Could you check a few things on this model? Use its own coordinates, in mm. A direction names the side the tool comes from. Round coordinates to 2 decimals unless told otherwise and drop trailing zeros. Write each loop counter-clockwise with the first axis right and the second up, starting at its lowest first coordinate (ties: lowest second). Pieces come first, ordered by that corner, then holes. Notation, with made-up numbers: M -27.5,77.5 L -16.5,77.5 A11 cw -16.5,92.5 Z; hole C 62.25,65 d2. An arc over 180 degrees is marked long. One line per item, written item: value. Start each with the question number.
(1) I want a section at C-C on z = 46.5. Please give me the cut outline in (x, y), and give its area (3 significant figures).
(2) Thinking about a two-plate mould opening in Y: for faces 1 (the face through (12.535, 4.207, 24.65)), 2 (the face through (60, 14, 25)), 3 (the face through (10, 39.879, 25)), which applies, released by +Y, released by -Y, zero draft, split by the parting line, or undercut?
(3) I want a section at B-B on x = 12. Please give me the cut outline in (y, z), and give its area (3 significant figures).
(4) Which directions (+Z, -Z, +X, -X, +Y, -Y) give clear straight access to the entire face, cutting with the end or side of a thin tool? Please do faces 4 (the face through (39.93, 34.845, 24.719)), 5 (the face through (7, 8.151, 25)), 6 (the face through (47.535, 4.404, 24.65)).
(5) I want a section at A-A on y = 36.5. Please give me the cut outline in (x, z).
(6) If I drill on L1, parallel to Y at x = 33, z = 6; L2, parallel to Y at x = 3.5, z = 32; L3, parallel to X at y = 32, z = 37, over which ranges is the centre line in solid material (lowest first)?
(7) I'm going to push flat-ended pins straight in: pin 1 Ø4 at (x, y) = (21, 23.5) entering from -Z; pin 2 Ø12 at (y, z) = (24.5, 20.5) entering from +X; pin 3 Ø3 at (x, y) = (11, 23.5) entering from +Z; pin 4 Ø8 at (x, z) = (10, 20) entering from +Y. Where does each tip first touch, or does it pass through?
(8) I want a section at D-D on z = 12. Please give me the cut outline in (x, y), and give its area (3 significant figures).
Autodesk Fusion 360 part; units mm, degrees
sketch "Front View" plane through (0, 0, 0) normal (0, 0, 1) x (1, 0, 0)
  line L0 (0, 19.879) -> (0, 8.1508)
  line L1 (0, 8.1508) -> (15, 8.1508)
  line L2 (15, 8.1508) -> (10, 0.1508)
  line L3 (10, 0.1508) -> (50, 0.1508)
  line L4 (50, 0.1508) -> (45, 8.777)
  line L5 (45, 8.777) -> (60, 8.777)
  line L6 (60, 8.777) -> (60, 19.879)
  line L7 (60, 19.879) -> (0, 19.879)
  line L8 (5, 19.879) -> (5, 39.879)
  line L9 (5, 39.879) -> (15, 39.879)
  line L10 (25, 29.879) -> (35, 29.879)
  line L11 (45, 39.953) -> (55, 39.953)
  line L12 (55, 39.953) -> (55, 19.879)
  line L13 (15, 39.879) -> (25, 29.879)
  line L14 (35, 29.879) -> (45, 39.953)
  dimension "d1" = 8
  dimension "d2" = 11.7282
  dimension "d3" = 10
  dimension "d4" = 40
  dimension "d5" = 30
  dimension "d6" = 20
  dimension "d7" = 60
  dimension "d8" = 5
  dimension "d9" = 5
  dimension "d10" = 10
  dimension "d11" = 10
  dimension "d12" = 10
  dimension "d13" = 10
  dimension "d14" = 10
  dimension "d16" = 10
  dimension "d17" = 5
extrude "Extrude1" add sketch "Front View" along normal blind 50 contours L0 L1 L2 L3 L4 L5 L6 L7
sketch "Side View" plane through (0, 0, 0) normal (1, 0, 0) x (0, 0, -1)
  line L0 (-50.0346, 20.0445) -> (-40.0346, 38.5513)
  line L1 (-27, 38.5513) -> (-40.0346, 38.5513)
  line L2 (-27, 38.5513) -> (-10.0346, 38.5513)
  line L3 (-0.0346, 20.0445) -> (-10.0346, 38.5513)
  line L4 (-50.0346, 20.0445) -> (-0.0346, 20.0445)
  line L5 (-50.0346, 20.0445) -> (-0.0346, 20.0445)
  line L6 (-0.0346, 20.0445) -> (-0.0346, 8.0445)
  line L7 (-0.0346, 8.0445) -> (-50.0346, 8.0445)
  line L8 (-50.0346, 8.0445) -> (-50.0346, 20.0445)
  line L9 (-50.0346, 8.0445) -> (-0.0346, 8.0445)
  line L10 (-0.0346, 8.0445) -> (-0.0346, 0.0445)
  line L11 (-0.0346, 0.0445) -> (-50.0346, 0.0445)
  line L12 (-50.0346, 0.0445) -> (-50.0346, 8.0445)
  dimension "d32" = 12
  dimension "d33" = 50
  dimension "d34" = 50
  dimension "d35" = 8
  dimension "d36" = 30
  dimension "d37" = 10
  dimension "d38" = 10
extrude "Extrude4" add sketch "Front View" along normal blind 50 contours L7 L8 L9 L10 L11 L12 L13 L14
chamfer "Chamfer2" distance 20 distance2 10 1 edges at (50, 39.953, 0) measured on face at (28.3333, 15.6022, 0)
chamfer "Chamfer3" distance 20 distance2 10 1 edges at (50, 39.953, 50) measured on face at (28.3333, 15.6022, 50)
extrude "Extrude3" [suppressed]
Found:
1. outline: M 0,8.15 L 15,8.15 L 10,0.15 L 50,0.15 L 45,8.78 L 60,8.78 L 60,19.88 L 55,19.88 L 55,26.95 L 5,26.95 L 5,19.88 L 0,19.88 Z
1. area: 1,330 mm²
2. face 1: undercut
2. face 2: zero draft
2. face 3: released by +Y
3. outline: M 0.15,0 L 3.35,0 L 3.35,50 L 0.15,50 Z; M 8.15,0 L 19.95,0 L 39.88,9.96 L 39.88,40.04 L 19.95,50 L 8.15,50 Z
3. area: 1,550 mm²
4. face 4: +Z, -Z, +Y
4. face 5: +Z, -Z, -X
4. face 6: +Z, -Z, +X
5. outline: M 5,8.27 L 18.38,8.27 L 18.38,41.73 L 5,41.73 Z; M 41.57,8.27 L 55,8.27 L 55,41.73 L 41.57,41.73 Z
6. L1: y = 0.15 to 29.88
6. L2: y = 8.15 to 19.88
6. L3: x = 5 to 22.88, 37.11 to 55
7. pin 1: stops at z = 0.77
7. pin 2: stops at x = 60
7. pin 3: stops at z = 48.98
7. pin 4: stops at y = 39.88
8. outline: M 0,8.15 L 15,8.15 L 10,0.15 L 50,0.15 L 45,8.78 L 60,8.78 L 60,19.88 L 55,19.88 L 55,39.95 L 45,39.95 L 35,29.88 L 25,29.88 L 15,39.88 L 5,39.88 L 5,19.88 L 0,19.88 Z
8. area: 1,780 mm²
